The listing builds one solid part. Answer for the finished solid, in the listing's coordinates (mm). Round coordinates to 2 decimals unless told otherwise and drop trailing zeros. Write each loop counter-clockwise with the first axis right and the second up, starting at its lowest first coordinate (ties: lowest second). Pieces come first, ordered by that corner, then holes.
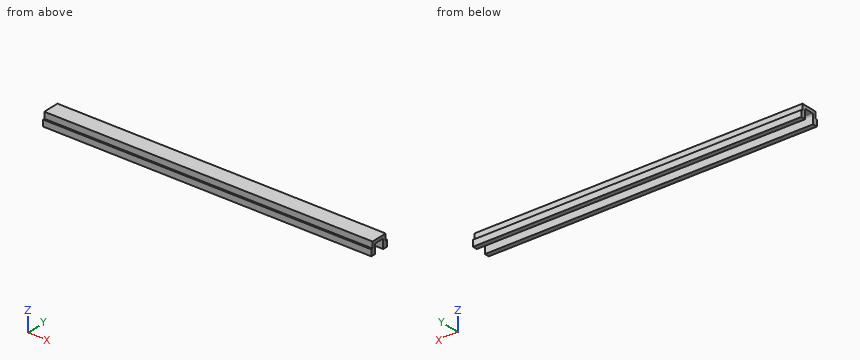
from build123d import *

# Parameters (mm, degrees)
F0_W          = 104
F0_H          = 5.2
F1_DEPTH      = 3
F0_H_2        = 2
F2_DEPTH      = 1
F2_DEPTH_BACK = 1
F3_W          = 1.5
F3_H          = 2
F4_DEPTH      = 104


with BuildPart() as f1:
    # F0 (on Top) → F1 (new body)
    with BuildSketch(Plane.XY):
        with Locations((7.6501901746, -8.5250005215)):
            Rectangle(F0_W, F0_H)
    extrude(amount=F1_DEPTH)

    # F0 (on Top) → F2 (join, two sides)
    with BuildSketch(Plane.XY) as f2_sk:
        with Locations((7.6501901746, -4.9250005215)):
            Rectangle(F0_W, F0_H_2)
        with Locations((7.6501901746, -8.5250005215)):
            Rectangle(F0_W, F0_H)
        with Locations((7.6501901746, -12.1250005215)):
            Rectangle(F0_W, F0_H_2)
    extrude(amount=-F2_DEPTH)
    extrude(f2_sk.sketch, amount=F2_DEPTH_BACK)

    # F3 (on face) → F4 (cut)
    with BuildSketch(Plane.YZ.offset(59.6501901746)):
        with Locations((-12.3750005215, 0)):
            Rectangle(F3_W, F3_H)
        with BuildLine():
            Line((-10.1250005215, -1), (-6.9250005215, -1))
            Line((-6.9250005215, -1), (-6.9250005215, 1.6))
            ThreePointArc((-6.9250005215, 1.6), (-7.0421578091, 1.8828427125), (-7.3250005215, 2))
            Line((-7.3250005215, 2), (-9.7250005215, 2))
            ThreePointArc((-9.7250005215, 2), (-10.007843234, 1.8828427125), (-10.1250005215, 1.6))
            Line((-10.1250005215, 1.6), (-10.1250005215, -1))
        make_face()
        with Locations((-4.6750005215, 0)):
            Rectangle(F3_W, F3_H)
    extrude(amount=-F4_DEPTH, mode=Mode.SUBTRACT)


solid = f1.part
1. Straight lines are drawn through the part: line 1 along Y through (x, z) = (41, 0.4) (3 decimals); line 2 along Y through (x, z) = (44, 1.65) (3 decimals); line 3 along Z through (x, y) = (51.5, -8.5). For each, find the intervals that lie inside material, in ascending order.
Geometry says:
line 1: y = -11.625 to -10.125, -6.925 to -5.425
line 2: y = -11.125 to -10.122, -6.928 to -5.925
line 3: z = 2 to 3
2. Given pin 1 (1.6 mm diameter, centred on x = 25.5, z = 2, fed in from -Y) (3 decimals); pin 2 (0.6 mm diameter, centred on x = 8.5, y = -11.5, fed in from +Z); pin 3 (1.9 mm diameter, centred on x = -11.5, y = -8, fed in from -Z), each flat-ended and moving along its own axis, determine where each tip first touches the part or whether it passes through.
Geometry says:
pin 1: stops at y = -11.125
pin 2: stops at z = 1
pin 3: stops at z = 1.89
3. Section C-C on y = -8.5 is taken. Determine the outline of the cut face in (x, z).
Geometry says:
outline: (-44.35, 2) - (59.65, 2) - (59.65, 3) - (-44.35, 3) - close
4. Section A-A on z = 0.3 is taken. Determine the outline of the cut face in (x, y) (3 decimals).
Geometry says:
outline: (-44.35, -11.625) - (59.65, -11.625) - (59.65, -10.125) - (-44.35, -10.125) - close; (-44.35, -6.925) - (59.65, -6.925) - (59.65, -5.425) - (-44.35, -5.425) - close
5. Section B-B on x = -13 is taken. Determine the outline of the cut face in (y, z) (3 decimals), plus the area to 3 significant figures.
Geometry says:
outline: (-11.625, -1) - (-10.125, -1) - (-10.125, 1.6) arc R0.4 cw to (-9.725, 2) - (-7.325, 2) arc R0.4 cw to (-6.925, 1.6) - (-6.925, -1) - (-5.425, -1) - (-5.425, 1) - (-5.925, 1) - (-5.925, 3) - (-11.125, 3) - (-11.125, 1) - (-11.625, 1) - close
area: 13.3 mm2
